Geometry: final body of the model. Coordinates: model frame, mm. Face numbers are marked on the shaded views. A direction names the side the tool comes from. Give positions to 0.01 mm unless a question says otherwise; leave off trailing zeros. Loops run counter-clockwise (first coordinate to the right, second up) from the corner with the lowest first, then second, coordinate; pieces in that order, holes last. Notation, with made-up numbers: (20, 40.25) -> (68, 40.25) arc R29 cw to (68, 62.25) -> close; hole circle Ø2 at (3.5, 69). An arc over 180 degrees is marked (long way). Answer in a Markdown table with one row per item. Add a question column.
1) Draft query along Z for the marked faces 1, 2 and 3. Return one class per face: +Z half, -Z half, draft (parallel to the pull), parting line (faces both ways), or undercut.
2) Section query C-C (z = 4.75). Return the cut outline in (x, y), plus the area to 3 significant figures.
3) Line query: line 1 (Z direction, x = 0, y = 2.25) (3 decimals); line 2 (X direction, y = 2.25, z = 0) (3 decimals); line 3 (Z direction, x = -11.5, y = 1.5). Output: solid intervals per line, ascending. Write a range as from..to.
4) Section query B-B (y = 2). Return the cut outline in (x, z) (3 decimals), plus the area to 3 significant figures.
5) First-contact query: P1, Ø3.5, axis at x = -10.5, y = 3.5, coming from the -Z side; P2, Ø2.5, axis at x = -11.5, y = 3, coming from the +Z side. Flat tips, straight axial feed; report the tip coordinate or a pass-through.
6) Section query D-D (z = 0). Return the cut outline in (x, y) (3 decimals), plus the area to 3 significant figures.
7) Access query for the marked faces 4 and 5. Directions: +Z, -Z, +X, -X, +Y, -Y. A direction counts if a zero-diameter tool reaches every point of the face in a straight line with its end or side. Return the directions, or none.
8) Section query A-A (x = 0). Return the cut outline in (y, z) (3 decimals).
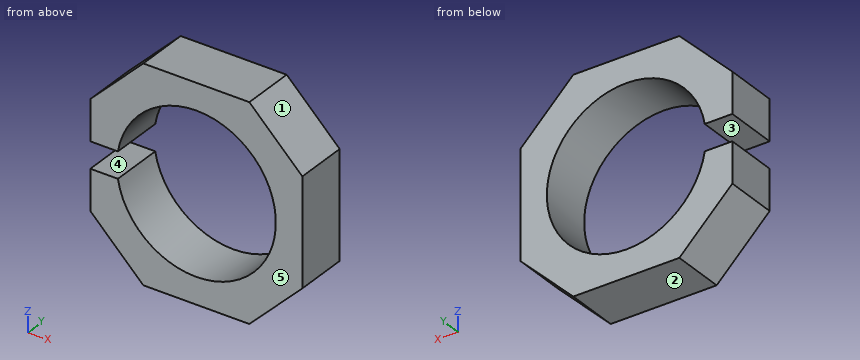
```python
from build123d import *

# Parameters (mm, degrees)
F0_W     = 25.4
F0_H     = 25.4
F1_DEPTH = 6.35
F2_R     = 9.525
F3_DEPTH = 6.35
F5_DEPTH = 6.35
F6_W     = 15.854515
F6_H     = 3.134032
F7_DEPTH = 6.35


with BuildPart() as f1:
    # F0 (on Front) → F1 (new body)
    with BuildSketch(Plane.XZ):
        Rectangle(F0_W, F0_H)
    extrude(amount=-F1_DEPTH)

    # F2 (on face) → F3 (cut)
    with BuildSketch(Plane.XZ):
        Circle(F2_R)
    extrude(amount=-F3_DEPTH, mode=Mode.SUBTRACT)

    # F4 (on Front) → F5 (cut)
    with BuildSketch(Plane.XZ):
        Polygon((12.761054, 6.350294), (12.7, 12.7), (6.35, 12.7), align=None)
        Polygon((-6.35, 12.7), (-12.7, 12.7), (-12.761054, 6.350294), align=None)
        Polygon((-12.761054, -6.350294), (-12.7, -12.7), (-6.35, -12.7), align=None)
        Polygon((6.35, -12.7), (12.7, -12.7), (12.761054, -6.350294), align=None)
    extrude(amount=-F5_DEPTH, mode=Mode.SUBTRACT)

    # F6 (on Front) → F7 (cut)
    with BuildSketch(Plane.XZ):
        with Locations((-14.840564, 0)):
            Rectangle(F6_W, F6_H)
    extrude(amount=-F7_DEPTH, mode=Mode.SUBTRACT)


solid = f1.part
```
Evaluation:
| question | item | result |
|---|---|---|
| 1 | face 1 | +Z half |
| 1 | face 2 | -Z half |
| 1 | face 3 | undercut |
| 2 | outline | (-12.7, 0) -> (-8.26, 0) -> (-8.26, 6.35) -> (-12.7, 6.35) -> close; (8.26, 0) -> (12.7, 0) -> (12.7, 6.35) -> (8.26, 6.35) -> close |
| 2 | area | 56.4 mm² |
| 3 | line 1 | -12.7..-9.525, 9.525..12.7 |
| 3 | line 2 | 9.525..12.7 |
| 3 | line 3 | -7.6..-1.57, 1.57..7.6 |
| 4 | outline | (-12.7, -6.411) -> (-6.35, -12.7) -> (6.35, -12.7) -> (12.7, -6.411) -> (12.7, 6.411) -> (6.35, 12.7) -> (-6.35, 12.7) -> (-12.7, 6.411) -> (-12.7, 1.567) -> (-9.395, 1.567) arc R9.525 cw (long way) to (-9.395, -1.567) -> (-12.7, -1.567) -> close |
| 4 | area | 270 mm² |
| 5 | P1 | z = -10.32 |
| 5 | P2 | z = 8.84 |
| 6 | outline | (9.525, 0) -> (12.7, 0) -> (12.7, 6.35) -> (9.525, 6.35) -> close |
| 6 | area | 20.2 mm² |
| 7 | face 4 | -X, +Y, -Y |
| 7 | face 5 | +Z, -Z, +X, -X, -Y |
| 8 | outline | (0, -12.7) -> (6.35, -12.7) -> (6.35, -9.525) -> (0, -9.525) -> close; (0, 9.525) -> (6.35, 9.525) -> (6.35, 12.7) -> (0, 12.7) -> close |
